Design review of the part built by this model. Coordinates are the model's own, in mm. Face numbers are marked on the shaded views. Round coordinates to 2 decimals unless told otherwise and drop trailing zeros. Loops run counter-clockwise (first coordinate to the right, second up) from the corner with the lowest first, then second, coordinate; pieces in that order, holes last. Notation, with made-up numbers: M -28.75,-14.5 L 2.25,-14.5 A22 ccw 2.25,6.5 Z; hole C -27.5,13 d4. An arc over 180 degrees is marked long. Use a Markdown table: item, result.
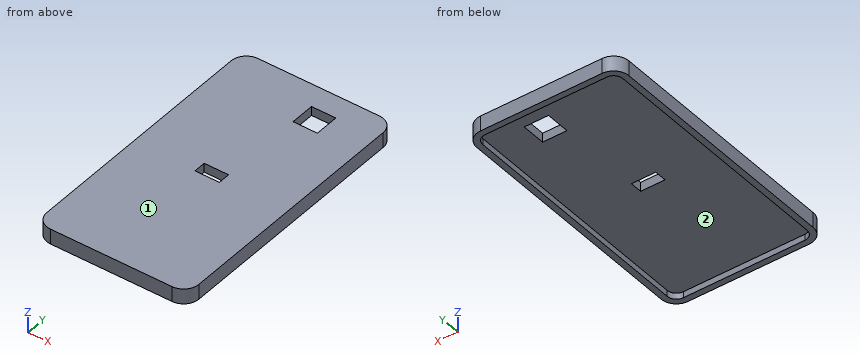
from build123d import *

# Parameters (mm, degrees)
SKETCH2_W           = 63.5
SKETCH2_H           = 114.3
BOSS_EXTRUDE1_DEPTH = 6.35
FILLET1_R           = 6.35
CUT_EXTRUDE2_DEPTH  = 2.54
SKETCH8_W           = 10.16
SKETCH8_H           = 10.16
CUT_EXTRUDE3_DEPTH  = 131.81
SKETCH7_W           = 10.16
SKETCH7_H           = 5.08
CUT_EXTRUDE4_DEPTH  = 131.81


with BuildPart() as part:
    # Sketch2 → Boss-Extrude1 (new body)
    with BuildSketch(Plane.XY):
        with Locations((31.75, -57.15)):
            Rectangle(SKETCH2_W, SKETCH2_H)
    extrude(amount=BOSS_EXTRUDE1_DEPTH)

    # Fillet1
    fillet1_edges = [part.edges().sort_by_distance(p)[0] for p in [
        (0, 0, 3.175),
        (63.5, 0, 3.175),
        (63.5, -114.3, 3.175),
        (0, -114.3, 3.175),
    ]]
    fillet(fillet1_edges, radius=FILLET1_R)

    # Sketch5 → Cut-Extrude2 (cut)
    with BuildSketch(Plane(origin=(0, 0, 0), x_dir=(-1, 0, 0), z_dir=(0, 0, -1))):
        with BuildLine():
            Line((-60.96, -6.453652416), (-60.96, -107.95))
            ThreePointArc((-60.96, -107.95), (-59.844076836, -110.644076836), (-57.15, -111.76))
            Line((-57.15, -111.76), (-6.35, -111.76))
            ThreePointArc((-6.35, -111.76), (-3.655923164, -110.644076836), (-2.54, -107.95))
            Line((-2.54, -107.95), (-2.54, -6.35))
            ThreePointArc((-2.54, -6.35), (-3.655923164, -3.655923164), (-6.35, -2.54))
            Line((-6.35, -2.54), (-57.15, -2.54))
            ThreePointArc((-57.15, -2.54), (-59.881396091, -3.692317076), (-60.96, -6.453652416))
        make_face()
    extrude(amount=-CUT_EXTRUDE2_DEPTH, mode=Mode.SUBTRACT)

    # Sketch8 → Cut-Extrude3 (cut, through all)
    with BuildSketch(Plane(origin=(0, 0, 2.54), x_dir=(-1, 0, 0), z_dir=(0, 0, -1))):
        with Locations((-41.148, -14.732)):
            Rectangle(SKETCH8_W, SKETCH8_H)
    extrude(amount=-CUT_EXTRUDE3_DEPTH, mode=Mode.SUBTRACT)

    # Sketch7 → Cut-Extrude4 (cut, through all)
    with BuildSketch(Plane(origin=(0, 0, 2.54), x_dir=(-1, 0, 0), z_dir=(0, 0, -1))):
        with Locations((-30.988, -57.912)):
            Rectangle(SKETCH7_W, SKETCH7_H)
    extrude(amount=-CUT_EXTRUDE4_DEPTH, mode=Mode.SUBTRACT)


solid = part.part
1. Take a section at B-B on x = 41. Give the boundary of the cut face in (y, z), and give its area (3 significant figures).
Check values:
| item | result |
|---|---|
| outline | M -114.3,0 L -111.76,0 L -111.76,2.54 L -19.81,2.54 L -19.81,6.35 L -114.3,6.35 Z; M -9.65,2.54 L -2.54,2.54 L -2.54,0 L 0,0 L 0,6.35 L -9.65,6.35 Z |
| area | 410 mm² |
2. Take a section at C-C on z = 1.5. Give the boundary of the cut face in (x, y).
Check values:
| item | result |
|---|---|
| outline | M 0,-107.95 A6.35 ccw 6.35,-114.3 L 57.15,-114.3 A6.35 ccw 63.5,-107.95 L 63.5,-6.35 A6.35 ccw 57.15,0 L 6.35,0 A6.35 ccw 0,-6.35 Z; hole M 2.54,-107.95 A3.81 ccw 6.35,-111.76 L 57.15,-111.76 A3.81 ccw 60.96,-107.95 L 60.96,-6.45 A3.81 ccw 57.15,-2.54 L 6.35,-2.54 A3.81 ccw 2.54,-6.35 Z |
3. Take a section at A-A on y = -16. Give the boundary of the cut face in (x, z), and give its area (3 significant figures).
Check values:
| item | result |
|---|---|
| outline | M 0,0 L 2.54,0 L 2.54,2.54 L 36.07,2.54 L 36.07,6.35 L 0,6.35 Z; M 46.23,2.54 L 60.96,2.54 L 60.96,0 L 63.5,0 L 63.5,6.35 L 46.23,6.35 Z |
| area | 216 mm² |
4. Insertion check: pin 1 (10 mm diameter, centred on x = 21, y = -11.5, fed in from -Z). The pin has a flat end and moves straight along its axis. Give the tip position at first contact, or say it passes through.
Check values:
| item | result |
|---|---|
| pin 1 | stops at z = 2.54 |
5. The part is to be moulded in two halves that separate along X. For the marked faces 1 and 2, say which applies: pulls with the +X half, pulls with the -X half, needs draft (parallel to the pull), parting line crosses it, or undercut.
Check values:
| item | result |
|---|---|
| face 1 | needs draft |
| face 2 | undercut |
6. Take a section at D-D on x = 12.5. Give the boundary of the cut face in (y, z).
Check values:
| item | result |
|---|---|
| outline | M -114.3,0 L -111.76,0 L -111.76,2.54 L -2.54,2.54 L -2.54,0 L 0,0 L 0,6.35 L -114.3,6.35 Z |
7. Wall thickness on line 1 along X through (y, z) = (-12, 3.25); line 2 along Y through (x, z) = (36.5, 1); line 3 along X through (y, z) = (-94, 2.5): over which ranges is each line inside the solid? List them lowest first. Write a range as from..to.
Check values:
| item | result |
|---|---|
| line 1 | x = 0..36.07, 46.23..63.5 |
| line 2 | y = -114.3..-111.76, -2.54..0 |
| line 3 | x = 0..2.54, 60.96..63.5 |
